Work out the finished part from the listing and answer in its coordinate system (mm). A direction names the side the tool comes from. Give positions to 0.01 mm unless a question says otherwise; leave off trailing zeros. Order: outer loops, then holes, each group sorted by start corner. A loop starts at its lowest first (then second) coordinate and runs counter-clockwise, first axis right, second up.
```python
from build123d import *

# Parameters (mm, degrees)
CUT_EXTRUDE1_REACH = 73.652


with BuildPart() as part:
    # Sketch1 → Revolve1 (revolve)
    with BuildSketch(Plane(origin=(0, 0, 0), x_dir=(1, 0, 0), z_dir=(0, 1, 0))):
        with BuildLine():
            Line((0, 70.09), (4.39217757, 70.09))
            ThreePointArc((4.39217757, 70.09), (4.487086316, 70.066046386), (4.559260987, 69.9999233))
            Line((4.559260987, 69.9999233), (5.440739013, 68.6600767))
            ThreePointArc((5.440739013, 68.6600767), (5.512913684, 68.593953614), (5.60782243, 68.57))
            Line((5.60782243, 68.57), (6.955, 68.57))
            Line((6.955, 68.57), (6.955, 68.67))
            Line((6.955, 68.67), (7.745, 68.67))
            Line((7.745, 68.67), (7.745, 68.97))
            Line((7.745, 68.97), (8.1, 68.97))
            Line((8.1, 68.97), (8.1, 69.15596492))
            ThreePointArc((8.1, 69.15596492), (8.127103293, 69.256497147), (8.201067285, 69.32978183))
            ThreePointArc((8.201067285, 69.32978183), (9.040599123, 69.672998391), (9.94, 69.79))
            ThreePointArc((9.94, 69.79), (10.350121933, 69.620121933), (10.52, 69.21))
            Line((10.52, 69.21), (10.52, 0.4))
            ThreePointArc((10.52, 0.4), (10.402842712, 0.117157288), (10.12, 0))
            Line((10.12, 0), (0, 0))
            Line((0, 0), (0, 68.27))
            Line((0, 68.27), (5.338266355, 68.27))
            Line((5.338266355, 68.27), (4.338266355, 69.79))
            Line((4.338266355, 69.79), (0, 69.79))
            Line((0, 69.79), (0, 70.09))
        make_face()
    revolve(axis=Axis((0, 0, 0), (0, 0, -1)))

    # Cut-Extrude1: up to this face of the body (flat: up to its plane)
    cut_extrude1_end = Plane(part.part.faces().sort_by_distance((0, 0, -68.27))[0])
    # Sketch2 → Cut-Extrude1 (cut, up to the picked face)
    with BuildSketch(Plane(origin=(0, 0, -70.09), x_dir=(-1, 0, 0), z_dir=(0, 0, -1)), mode=Mode.PRIVATE) as cut_extrude1_sk1:
        with BuildLine():
            ThreePointArc((5.588090856, -0.470013816), (4.856516684, 2.803911215), (2.387001523, 5.074435548))
            ThreePointArc((2.387001523, 5.074435548), (1.65, 4.808984945), (1.915450603, 4.071983422))
            ThreePointArc((1.915450603, 4.071983422), (3.897114317, 2.25), (4.484166389, -0.377162829))
            ThreePointArc((4.484166389, -0.377162829), (4.989703129, -0.975550556), (5.588090856, -0.470013816))
        make_face()
    cut_extrude1_tool1 = split(extrude(cut_extrude1_sk1.sketch, amount=-CUT_EXTRUDE1_REACH, mode=Mode.PRIVATE), bisect_by=cut_extrude1_end, keep=Keep.BOTH, mode=Mode.PRIVATE)
    # Sketch2 → Cut-Extrude1 (cut, up to the picked face)
    with BuildSketch(Plane(origin=(0, 0, -70.09), x_dir=(-1, 0, 0), z_dir=(0, 0, -1)), mode=Mode.PRIVATE) as cut_extrude1_sk2:
        with BuildLine():
            ThreePointArc((-3.201089333, -4.604421732), (0, -5.60782243), (3.201089333, -4.604421732))
            ThreePointArc((3.201089333, -4.604421732), (3.339703129, -3.833434389), (2.568715786, -3.694820593))
            ThreePointArc((2.568715786, -3.694820593), (0, -4.5), (-2.568715786, -3.694820593))
            ThreePointArc((-2.568715786, -3.694820593), (-3.339703129, -3.833434389), (-3.201089333, -4.604421732))
        make_face()
    cut_extrude1_tool2 = split(extrude(cut_extrude1_sk2.sketch, amount=-CUT_EXTRUDE1_REACH, mode=Mode.PRIVATE), bisect_by=cut_extrude1_end, keep=Keep.BOTH, mode=Mode.PRIVATE)
    # Sketch2 → Cut-Extrude1 (cut, up to the picked face)
    with BuildSketch(Plane(origin=(0, 0, -70.09), x_dir=(-1, 0, 0), z_dir=(0, 0, -1)), mode=Mode.PRIVATE) as cut_extrude1_sk3:
        with BuildLine():
            ThreePointArc((-2.387001523, 5.074435548), (-4.856516684, 2.803911215), (-5.588090856, -0.470013816))
            ThreePointArc((-5.588090856, -0.470013816), (-4.989703129, -0.975550556), (-4.484166389, -0.377162829))
            ThreePointArc((-4.484166389, -0.377162829), (-3.897114317, 2.25), (-1.915450603, 4.071983422))
            ThreePointArc((-1.915450603, 4.071983422), (-1.65, 4.808984945), (-2.387001523, 5.074435548))
        make_face()
    cut_extrude1_tool3 = split(extrude(cut_extrude1_sk3.sketch, amount=-CUT_EXTRUDE1_REACH, mode=Mode.PRIVATE), bisect_by=cut_extrude1_end, keep=Keep.BOTH, mode=Mode.PRIVATE)
    add(cut_extrude1_tool1.solids().sort_by(Axis((-4.048123, 2.337185, -70.09), (0, 0, 1)))[0], mode=Mode.SUBTRACT)
    add(cut_extrude1_tool2.solids().sort_by(Axis((0, -4.67437, -70.09), (0, 0, 1)))[0], mode=Mode.SUBTRACT)
    add(cut_extrude1_tool3.solids().sort_by(Axis((4.048123, 2.337185, -70.09), (0, 0, 1)))[0], mode=Mode.SUBTRACT)


solid = part.part
```
1. Given P1, Ø3, axis at y = -3.5, z = -16.5, coming from the -X side, flat-ended and moving along its own axis, determine where the tip first touches the part or whether it passes through.
Findings below:
P1: stops at x = -10.33
2. The part is cut by section B-B (z = -41.5). Write down the section's boundary in (x, y).
Findings below:
outline: circle Ø21.04 at (0, 0)
3. Which of the six approach directions +Z, -Z, +X, -X, +Y, -Y give full straight-line access (tool end or side, diameter ignored) to faces 4 (the face through (0, 0, -70.09)), 5 (the face through (6, -4, -68.67)), 6 (the face through (0, 0, -68.27))?
Findings below:
face 4: -Z, +X, -X, +Y, -Y
face 5: -Z
face 6: none
4. Straight lines are drawn through the part: probe 1 along Z at (x, y) = (-2.75, 1.5); probe 2 along X at (y, z) = (0, -69.05); probe 3 along Y at (x, z) = (0, -69.1). For each, find the intervals that lie inside material, in ascending order.
Findings below:
probe 1: z = -70.09 to -69.79, -68.27 to 0
probe 2: x = -10.52 to -8.1, 8.1 to 10.52
probe 3: y = -10.52 to -8.1, 4.79 to 5.15, 8.1 to 10.52
5. The mould has two halves that part along X. Classify faces 1 (the face through (-1.01, -7.68, -68.82)), 2 (the face through (0, 0, 0)), 3 (the face through (-2.28, 10.27, -34.32)): pulls with the +X half, pulls with the -X half, needs draft (parallel to the pull), parting line crosses it, or undercut.
Findings below:
face 1: undercut
face 2: needs draft
face 3: parting line crosses it
